Source: three-view drawing plus pictorial views. Frame: mm from the lowest corner of the part. Coordinates: 2 decimals unless noted, no trailing zeros. Write each loop counter-clockwise with the first axis right and the second up, starting at its lowest first coordinate (ties: lowest second). Pieces come first, ordered by that corner, then holes. Notation, with made-up numbers: (-40, 63.25) - (3, 63.25) arc R19 ccw to (3, 87.25) - close; hole circle Ø5 at (52, -21). An arc over 180 degrees is marked (long way). Put each result on its own line as item: value.
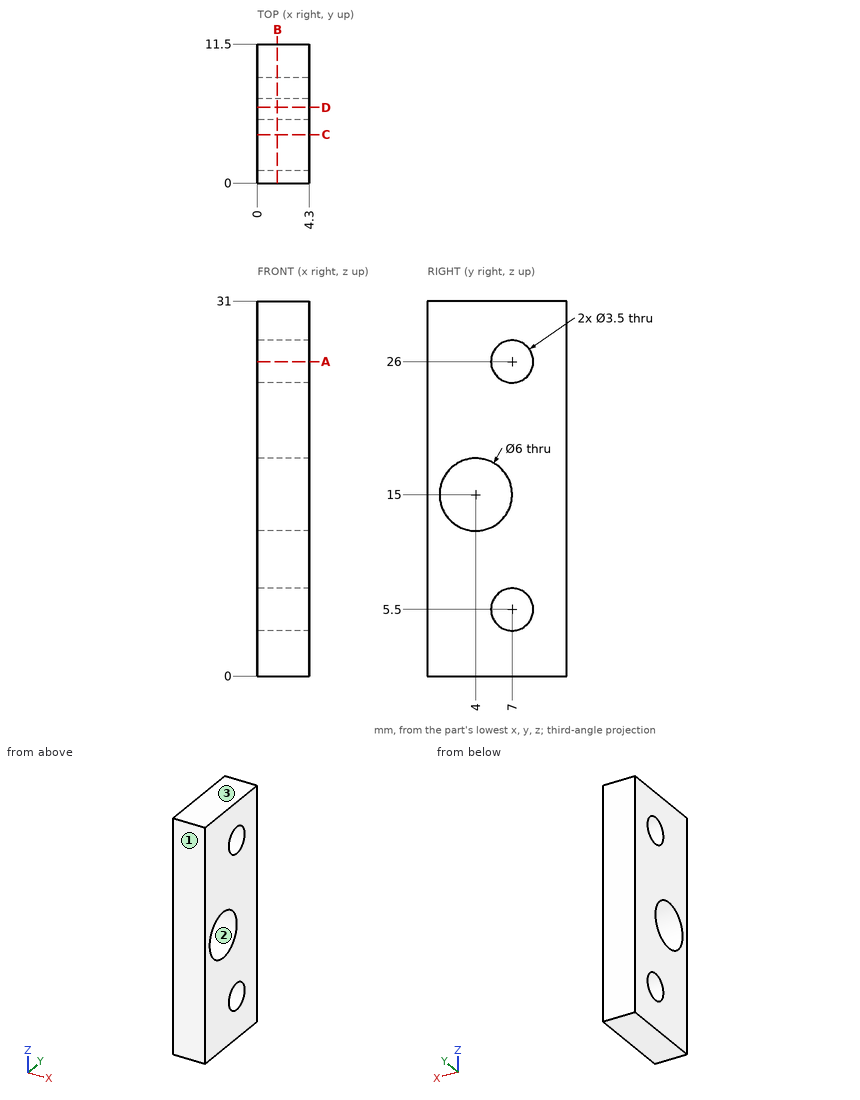
1. Ray query, probe 1 along Z at (x, y) = (2.2, 5.75); probe 2 along Z at (x, y) = (2.55, 8.5); probe 3 along Z at (x, y) = (1.9, 8.25). Return the intervals inside material, ascending. Write a range as from..to.
Answer below:
probe 1: z = 0..4.28, 6.72..12.56, 17.44..24.78, 27.22..31
probe 2: z = 0..4.6, 6.4..25.1, 26.9..31
probe 3: z = 0..4.28, 6.72..24.78, 27.22..31
2. Section query C-C (y = 4). Return loops of the section in (x, z).
Answer below:
outline: (0, 0) - (4.3, 0) - (4.3, 12) - (0, 12) - close; (0, 18) - (4.3, 18) - (4.3, 31) - (0, 31) - close
3. Pin query (flat end, axial travel): pin 1 Ø4.5 at (y, z) = (7, 5.5) entering from +X. Return the tip coordinate at first contact, or that it passes through.
Answer below:
pin 1: stops at x = 4.3
4. Section query D-D (y = 6.25). Return loops of the section in (x, z).
Answer below:
outline: (0, 0) - (4.3, 0) - (4.3, 3.92) - (0, 3.92) - close; (0, 7.08) - (4.3, 7.08) - (4.3, 13.02) - (0, 13.02) - close; (0, 16.98) - (4.3, 16.98) - (4.3, 24.42) - (0, 24.42) - close; (0, 27.58) - (4.3, 27.58) - (4.3, 31) - (0, 31) - close
5. Mould query, pull axis Y, two halves, no side actions, for the marked faces 1, 2 and 3. Classes: +Y half, -Y half, draft (parallel to the pull), parting line (faces both ways), or undercut.
Answer below:
face 1: -Y half
face 2: undercut
face 3: draft
6. Section query A-A (z = 26). Return loops of the section in (x, y), then the cut area to 3 significant figures.
Answer below:
outline: (0, 0) - (4.3, 0) - (4.3, 5.25) - (0, 5.25) - close; (0, 8.75) - (4.3, 8.75) - (4.3, 11.5) - (0, 11.5) - close
area: 34.4 mm²
7. Section query B-B (x = 1.65). Return loops of the section in (y, z).
Answer below:
outline: (0, 0) - (11.5, 0) - (11.5, 31) - (0, 31) - close; hole circle Ø6 at (4, 15); hole circle Ø3.5 at (7, 5.5); hole circle Ø3.5 at (7, 26)
